from build123d import *

# Parameters (mm, degrees)
SKETCH1_W                      = 64
SKETCH1_H                      = 60
BASE_FLANGE1_DEPTH             = 2
EDGE_FLANGE1_STRIP_W           = 9.4732
EDGE_FLANGE1_STRIP_H           = 2
EDGE_FLANGE1_STRIP_CUT_DEPTH   = 60
EDGE_FLANGE1_STRIP_2_W         = 9.4732
EDGE_FLANGE1_STRIP_2_H         = 2
EDGE_FLANGE1_STRIP_CUT_2_DEPTH = 60
EDGE_FLANGE1_DEPTH             = 60
EDGE_FLANGE1_BEND_DEPTH        = 60
SKETCH12_W                     = 4
SKETCH12_H                     = 22
BOSS_EXTRUDE1_DEPTH            = 19
FILLET1_R                      = 2
FILLET1_OF_MIRROR1_R           = 2
F_6_0MM_DOWEL_HOLE1_D          = 6
F_6_0MM_DOWEL_HOLE1_DEPTH      = 12
F_6_0MM_DOWEL_HOLE1_TIP        = 1.802581857
CUT_EXTRUDE1_REACH             = 64.49
SKETCH19_R                     = 10
CIRPATTERN1_COUNT              = 3


# Sheet-metal steps are written as plain solids
with BuildPart() as part:
    # Sketch1 → Base-Flange1 (new body)
    with BuildSketch(Plane.XY):
        Rectangle(SKETCH1_W, SKETCH1_H)
    extrude(amount=-BASE_FLANGE1_DEPTH)

    # Edge-Flange1 strip (across the edge) → Edge-Flange1 strip cut (cut)
    with BuildSketch(Plane(origin=(-32, 30, 0), x_dir=(1, 0, 0), z_dir=(0, -1, 0))):
        with Locations((-4, -1)):
            Rectangle(EDGE_FLANGE1_STRIP_W, EDGE_FLANGE1_STRIP_H)
    extrude(amount=EDGE_FLANGE1_STRIP_CUT_DEPTH, mode=Mode.SUBTRACT)

    # Edge-Flange1 strip 2 (across the edge) → Edge-Flange1 strip cut 2 (cut)
    with BuildSketch(Plane(origin=(32, -30, 0), x_dir=(-1, 0, 0), z_dir=(0, 1, 0))):
        with Locations((-4, -1)):
            Rectangle(EDGE_FLANGE1_STRIP_2_W, EDGE_FLANGE1_STRIP_2_H)
    extrude(amount=EDGE_FLANGE1_STRIP_CUT_2_DEPTH, mode=Mode.SUBTRACT)

    # Edge-Flange1 section (across the edge) → Edge-Flange1 (add)
    with BuildSketch(Plane(origin=(-32, 30, 0), x_dir=(1, 0, 0), z_dir=(0, -1, 0))):
        with BuildLine():
            Line((-2, 0.7366), (-2, 14))
            Line((-2, 14), (0, 14))
            Line((0, 14), (0, 0.7366))
            ThreePointArc((0, 0.7366), (0.215745145, 0.215745145), (0.7366, 0))
            Line((0.7366, 0), (0.7366, -2))
            ThreePointArc((0.7366, -2), (-1.198468417, -1.198468417), (-2, 0.7366))
        make_face()
    extrude(amount=EDGE_FLANGE1_DEPTH)

    # Edge-Flange1 section 2 (across the edge) → Edge-Flange1 bend (add)
    with BuildSketch(Plane(origin=(32, -30, 0), x_dir=(-1, 0, 0), z_dir=(0, 1, 0))):
        with BuildLine():
            Line((-2, 0.7366), (-2, 14))
            Line((-2, 14), (0, 14))
            Line((0, 14), (0, 0.7366))
            ThreePointArc((0, 0.7366), (0.215745145, 0.215745145), (0.7366, 0))
            Line((0.7366, 0), (0.7366, -2))
            ThreePointArc((0.7366, -2), (-1.198468417, -1.198468417), (-2, 0.7366))
        make_face()
    extrude(amount=EDGE_FLANGE1_BEND_DEPTH)

    # Sketch12 → Boss-Extrude1 (add)
    with BuildSketch(Plane.ZY.offset(34)):
        with Locations((12, 0)):
            Rectangle(SKETCH12_W, SKETCH12_H)
    boss_extrude1 = extrude(amount=BOSS_EXTRUDE1_DEPTH)

    # Fillet1
    fillet1_edges = [part.edges().sort_by_distance(p)[0] for p in [
        (-53, 11, 12),
        (-53, -11, 12),
    ]]
    fillet(fillet1_edges, radius=FILLET1_R)

    # Mirror1: Boss-Extrude1 across plane
    add(boss_extrude1.mirror(Plane(origin=(0, 0, 0), x_dir=(0, 0, 1), z_dir=(1, 0, 0))))

    # Fillet1 of Mirror1
    fillet1_of_mirror1_edges = [part.edges().sort_by_distance(p)[0] for p in [
        (53, 11, 12),
        (53, -11, 12),
    ]]
    fillet(fillet1_of_mirror1_edges, radius=FILLET1_OF_MIRROR1_R)

    # Ø6.0mm Dowel Hole1
    with Locations(Plane(origin=(0, 0, 10), x_dir=(-1, 0, 0), z_dir=(0, 0, -1))):
        with Locations((-43, 0), (43, 0)):
            Hole(F_6_0MM_DOWEL_HOLE1_D / 2, depth=F_6_0MM_DOWEL_HOLE1_DEPTH)
            with Locations((0, 0, -(F_6_0MM_DOWEL_HOLE1_DEPTH + F_6_0MM_DOWEL_HOLE1_TIP / 2))):  # 118° drill point
                Cone(0, F_6_0MM_DOWEL_HOLE1_D / 2, F_6_0MM_DOWEL_HOLE1_TIP, mode=Mode.SUBTRACT)

    # Sketch19 → Cut-Extrude1 (cut, up to next)
    with BuildSketch(Plane.XY, mode=Mode.PRIVATE) as cut_extrude1_sk1:
        Circle(SKETCH19_R)
    cut_extrude1_tool1 = extrude(cut_extrude1_sk1.sketch, amount=-CUT_EXTRUDE1_REACH, mode=Mode.PRIVATE) & part.part
    add(cut_extrude1_tool1.solids().sort_by_distance((0, 0, 0))[0], mode=Mode.SUBTRACT)

    # Sketch20 → Ø3.0mm Dowel Hole1 (revolve, cut)
    with BuildSketch(Plane(origin=(0, 15, 0), x_dir=(0, -1, 0), z_dir=(1, 0, 0))):
        Polygon((0, 0), (0, 12.901290929), (1.5, 12), (1.5, 0), align=None)
    f_3_0mm_dowel_hole1 = revolve(axis=Axis((0, 15, 6.35), (0, 0, -1)), mode=Mode.SUBTRACT)

    # CirPattern1: Ø3.0mm Dowel Hole1 ×3 about axis
    cirpattern1_axis = Axis((0, 0, 0), (0, 0, 1))
    for i in range(1, CIRPATTERN1_COUNT):
        add(f_3_0mm_dowel_hole1.rotate(cirpattern1_axis, i * 360 / CIRPATTERN1_COUNT), mode=Mode.SUBTRACT)


solid = part.part
Work out the finished part from the listing and answer in its coordinate system (mm). A direction names the side the tool comes from. Coordinates: 2 decimals unless noted, no trailing zeros. Loops run counter-clockwise (first coordinate to the right, second up) from the corner with the lowest first, then second, coordinate; pieces in that order, holes last. Notation, with made-up numbers: (-14.5, 9.25) -> (19.5, 9.25) arc R26 ccw to (19.5, 31.25) -> close; hole circle Ø6 at (22, -21.5). An arc over 180 degrees is marked (long way). Write each question's results on one line, items separated by ' | '. Start each with the question number.
1) Consider line 1 along Y through (x, z) = (0, -1.15); line 2 along Y through (x, z) = (-43, 11.8); line 3 along X through (y, z) = (7.5, 9). Determine where each line is inside the solid, lowest interval first.
2) Find section C-C on y = 0. Determine the outline of the cut face in (x, z), then the cut area to 3 significant figures.
3) Flat-ended cylindrical pins translate along their axes: P1, Ø15, axis at x = 39, y = -1, coming from the -Z side; P2, Ø1.8, axis at x = 0, y = 15, coming from the -Z side; P3, Ø1.2, axis at x = -42, z = 11, coming from the -Y side; P4, Ø4, axis at y = 5.5, z = 0.5, coming from the -X side. Find the tip coordinate at first contact, or state that the pin passes through.
4) Find section A-A on x = 0. Determine the outline of the cut face in (y, z), then the cut area to 3 significant figures.
5) For faces 4 (the flat face through (-7.4, 7.1, 0)), 5 (the flat face through (-45, -3, 10)), 6 (the flat face through (42, 11, 12)), 7 (the flat face through (-38, 0, 14)), determine the directions among +Z, -Z, +X, -X, +Y, -Y from which every point of the face is accessible in a straight line to the end or side of a thin tool.
6) Find section B-B on x = -43. Determine the outline of the cut face in (y, z), then the cut area to 3 significant figures.
7) The mould has two halves that part along Y. Classify faces 1 (the flat face through (-42, 11, 12)), 2 (the cylindrical face through (33.177, -0.42, -1.22)), 3 (the cylindrical face through (-14.478, -7.305, -0.986)): pulls with the +Y half, pulls with the -Y half, needs draft (parallel to the pull), parting line crosses it, or undercut.
8) Find section D-D on z = 4. Determine the outline of the cut face in (x, y), then the cut area to 3 significant figures.
Response values:
1) line 1: y = -30 to -10, 10 to 13.5, 16.5 to 30 | line 2: y = -11 to -3, 3 to 11 | line 3: x = -34 to -32, 32 to 34
2) outline: (-53, 10) -> (-46, 10) -> (-46, 14) -> (-53, 14) -> close; (-40, 10) -> (-34, 10) -> (-34, 0.74) arc R2.74 ccw to (-31.26, -2) -> (-10, -2) -> (-10, 0) -> (-31.26, 0) arc R0.74 cw to (-32, 0.74) -> (-32, 14) -> (-40, 14) -> close; (10, -2) -> (31.26, -2) arc R2.74 ccw to (34, 0.74) -> (34, 10) -> (40, 10) -> (40, 14) -> (32, 14) -> (32, 0.74) arc R0.74 cw to (31.26, 0) -> (10, 0) -> close; (46, 10) -> (53, 10) -> (53, 14) -> (46, 14) -> close | area: 253 mm^2
3) P1: stops at z = -1.99 | P2: passes through | P3: stops at y = -11 | P4: stops at x = -34
4) outline: (-30, -2) -> (-10, -2) -> (-10, 0) -> (-30, 0) -> close; (10, -2) -> (13.5, -2) -> (13.5, 0) -> (10, 0) -> close; (16.5, -2) -> (30, -2) -> (30, 0) -> (16.5, 0) -> close | area: 74.0 mm^2
5) face 4: +Z, +Y, -Y | face 5: -Z, -X, +Y, -Y | face 6: +Z, -Z, +X, +Y | face 7: +Z, +X, -X, +Y, -Y
6) outline: (-11, 10) -> (-3, 10) -> (-3, 14) -> (-11, 14) -> close; (3, 10) -> (11, 10) -> (11, 14) -> (3, 14) -> close | area: 64.0 mm^2
7) face 1: pulls with the +Y half | face 2: needs draft | face 3: undercut
8) outline: (-34, -30) -> (-32, -30) -> (-32, 30) -> (-34, 30) -> close; (32, -30) -> (34, -30) -> (34, 30) -> (32, 30) -> close | area: 240 mm^2
